Geometry check sheet. Reference: the model listing, model coordinates, mm. Round coordinates to 2 decimals unless told otherwise and drop trailing zeros. Order: outer loops, then holes, each group sorted by start corner. A loop starts at its lowest first (then second) coordinate and runs counter-clockwise, first axis right, second up.
(1) Go/stop test with flat-tipped pins: pin 1 (3 mm diameter, centred on y = 3.5, z = -56.5, fed in from +X) (3 decimals); pin 2 (2 mm diameter, centred on x = -118, y = 5, fed in from +Z); pin 3 (5 mm diameter, centred on y = 3.5, z = 34.5, fed in from -X) (3 decimals). Record where each tip stops, or that it passes through.
(2) Material ranges on line 1 along X through (y, z) = (6, 124.5) (3 decimals); line 2 along Z through (x, y) = (44, 5.75); line 3 along Z through (x, y) = (145, 2), recorded low to high.
(3) Sectioned sample at C-C (x = 181). Record the boundary of the cut face in (y, z) (3 decimals), plus the area to 3 significant figures.
(4) Sectioned sample at A-A (z = -54). Record the boundary of the cut face in (x, y) (3 decimals), plus the area to 3 significant figures.
(5) Sectioned sample at B-B (y = 7.25). Record the boundary of the cut face in (x, z) (1 decimal), plus the area to 3 significant figures.
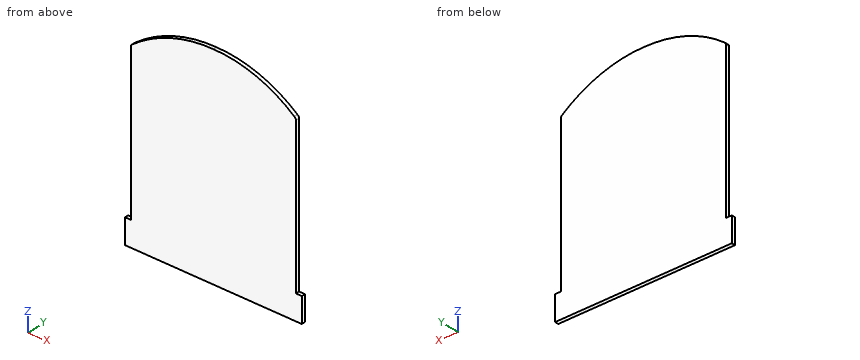
from build123d import *

# Parameters (mm, degrees)
BOSS_EXTRUDE3_DEPTH = 9.525


with BuildPart() as part:
    # Sketch1 → Boss-Extrude3 (new body)
    with BuildSketch(Plane(origin=(0, 0, 0), x_dir=(1, 0, 0), z_dir=(0, 1, 0))):
        with BuildLine():
            Line((-212.725, -228.6), (-212.725, 165.1))
            Line((-212.725, 165.1), (-227.9015, 165.1))
            Line((-227.9015, 165.1), (-227.9015, 228.6))
            Line((-227.9015, 228.6), (-212.725, 228.6))
            Line((-212.725, 228.6), (212.725, 228.6))
            Line((212.725, 228.6), (227.9015, 228.6))
            Line((227.9015, 228.6), (227.9015, 165.1))
            Line((227.9015, 165.1), (212.725, 165.1))
            Line((212.725, 165.1), (212.725, -228.6))
            ThreePointArc((212.725, -228.6), (211.576723559, -232.577910433), (208.573053823, -235.427520636))
            ThreePointArc((208.573053823, -235.427520636), (110.260259044, -288.46613371), (0, -306.3875))
            ThreePointArc((0, -306.3875), (-110.260259044, -288.46613371), (-208.573053823, -235.427520636))
            ThreePointArc((-208.573053823, -235.427520636), (-211.576723559, -232.577910433), (-212.725, -228.6))
        make_face()
    extrude(amount=BOSS_EXTRUDE3_DEPTH)


solid = part.part
Answer below:
1. pin 1: stops at x = 212.725
1. pin 2: stops at z = 286.09
1. pin 3: stops at x = -212.725
2. line 1: x = -212.725 to 212.725
2. line 2: z = -228.6 to 303.75
2. line 3: z = -228.6 to 274.44
3. outline: (0, -228.6) - (9.525, -228.6) - (9.525, 254.759) - (0, 254.759) - close
3. area: 4,600 mm2
4. outline: (-212.725, 0) - (212.725, 0) - (212.725, 9.525) - (-212.725, 9.525) - close
4. area: 4,050 mm2
5. outline: (-227.9, -228.6) - (227.9, -228.6) - (227.9, -165.1) - (212.7, -165.1) - (212.7, 228.6) arc R7.9 ccw to (208.6, 235.4) arc R336.4 ccw to (0, 306.4) arc R336.4 ccw to (-208.6, 235.4) arc R7.9 ccw to (-212.7, 228.6) - (-212.7, -165.1) - (-227.9, -165.1) - close
5. area: 220,000 mm2
